Input: part model. Units: mm. Frame: model coordinates. Face numbers are marked on the shaded views. A direction names the side the tool comes from. Give positions to 0.01 mm unless a question says otherwise; leave off trailing zeros. Order: outer loops, then holes, each group sorted by start corner. A loop starts at its lowest first (then second) coordinate and runs counter-clockwise, first axis right, second up. Notation, with made-up numbers: (6.25, 1.25) -> (50.25, 1.25) arc R29 cw to (50.25, 29.25) -> close; hole circle Ø5 at (-30, -14). An arc over 180 degrees is marked (long way). Use a Markdown table: item, result. Add a question column.
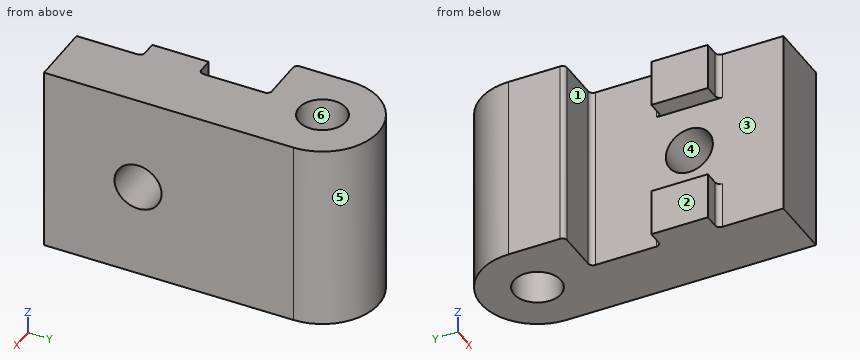
from build123d import *

# Parameters (mm, degrees)
SKETCH1_R           = 2.5
BOSS_EXTRUDE1_DEPTH = 20
SKETCH2_R           = 2.5
CUT_EXTRUDE1_DEPTH  = 20
SKETCH3_W           = 10
SKETCH3_H           = 6
CUT_EXTRUDE2_DEPTH  = 2
FILLET1_R           = 0.5
FILLET2_R           = 0.5


with BuildPart() as part:
    # Sketch1 → Boss-Extrude1 (new body)
    with BuildSketch(Plane.XY):
        with BuildLine():
            Line((6.3, -53.6), (6.3, -59.6))
            Line((6.3, -59.6), (7.3, -59.6))
            Line((7.3, -59.6), (8.3, -59.6))
            Line((8.3, -59.6), (8.3, -60.1))
            Line((8.3, -60.1), (8.3, -66.6))
            Line((8.3, -66.6), (15, -66.6))
            Line((15, -66.6), (15, -40.1))
            ThreePointArc((15, -40.1), (9, -34.1), (3, -40.1))
            Line((3, -40.1), (3, -46.1))
            Line((3, -46.1), (8.3, -46.1))
            Line((8.3, -46.1), (8.3, -46.6))
            Line((8.3, -46.6), (8.3, -53.1))
            Line((8.3, -53.1), (8.3, -53.6))
            Line((8.3, -53.6), (7.3, -53.6))
            Line((7.3, -53.6), (6.3, -53.6))
        make_face()
        with Locations((9, -40.1)):
            Circle(SKETCH1_R, mode=Mode.SUBTRACT)
    extrude(amount=BOSS_EXTRUDE1_DEPTH)

    # Sketch2 → Cut-Extrude1 (cut)
    with BuildSketch(Plane.ZY.offset(-6.3)):
        with Locations((10, -56.6)):
            Circle(SKETCH2_R)
    extrude(amount=-CUT_EXTRUDE1_DEPTH, mode=Mode.SUBTRACT)

    # Sketch3 → Cut-Extrude2 (cut)
    with BuildSketch(Plane.ZY.offset(-6.3)):
        with Locations((10, -56.6)):
            Rectangle(SKETCH3_W, SKETCH3_H)
    extrude(amount=-CUT_EXTRUDE2_DEPTH, mode=Mode.SUBTRACT)

    # Fillet1
    fillet1_edges = [part.edges().sort_by_distance(p)[0] for p in [
        (8.3, -46.1, 10),
        (3, -46.1, 10),
    ]]
    fillet(fillet1_edges, radius=FILLET1_R)

    # Fillet2
    fillet2_edges = [part.edges().sort_by_distance(p)[0] for p in [
        (8.3, -59.6, 17.5),
        (8.3, -53.6, 17.5),
        (8.3, -53.6, 2.5),
        (8.3, -59.6, 2.5),
    ]]
    fillet(fillet2_edges, radius=FILLET2_R)


solid = part.part
Q1. Section query A-A (x = 9). Return loops of the section in (y, z), plus the area to 3 significant figures.
Q2. Section query D-D (z = 17). Return loops of the section in (x, y), plus the area to 3 significant figures.
Q3. Section query B-B (z = 10). Return loops of the section in (x, y).
Q4. Access query for the marked faces 1, 2 and 3. Directions: +Z, -Z, +X, -X, +Y, -Y. A direction counts if a zero-diameter tool reaches every point of the face in a straight line with its end or side. Return the directions, or none.
Q5. Draft query along X for the marked faces 4, 5 and 6. Return one class per face: +X half, -X half, draft (parallel to the pull), parting line (faces both ways), or undercut.
Q6. First-contact query: pin 1 (1.5 mm diameter, centred on y = -58, z = 2, fed in from -X); pin 2 (1.7 mm diameter, centred on x = 7, z = 17, fed in from +Y); pin 3 (0.8 mm diameter, centred on x = 7.5, z = 16.5, fed in from -Y); pin 4 (4 mm diameter, centred on y = -56.6, z = 10, fed in from +X). Flat tips, straight axial feed; report the tip coordinate or a pass-through.
Q7. Ray query, line 1 (Y direction, x = 7.75, z = 1.75); line 2 (X direction, y = -40, z = 19); line 3 (Y direction, x = 9, z = 4.75). Return the intervals inside material, ascending.
Q8. Section query C-C (y = -56.6). Return loops of the section in (x, z), plus the area to 4 significant figures.
Solution:
| question | item | result |
|---|---|---|
| 1 | outline | (-66.6, 0) -> (-42.6, 0) -> (-42.6, 20) -> (-66.6, 20) -> close; (-37.6, 0) -> (-34.1, 0) -> (-34.1, 20) -> (-37.6, 20) -> close; hole circle Ø5 at (-56.6, 10) |
| 1 | area | 530 mm² |
| 2 | outline | (3, -45.6) arc R0.5 ccw to (3.5, -46.1) -> (7.8, -46.1) arc R0.5 cw to (8.3, -46.6) -> (8.3, -53.1) arc R0.5 cw to (7.8, -53.6) -> (6.3, -53.6) -> (6.3, -59.6) -> (7.8, -59.6) arc R0.5 cw to (8.3, -60.1) -> (8.3, -66.6) -> (15, -66.6) -> (15, -40.1) arc R6 ccw to (3, -40.1) -> close; hole circle Ø5 at (9, -40.1) |
| 2 | area | 258 mm² |
| 3 | outline | (3, -45.6) arc R0.5 ccw to (3.5, -46.1) -> (7.8, -46.1) arc R0.5 cw to (8.3, -46.6) -> (8.3, -54.1) -> (15, -54.1) -> (15, -40.1) arc R6 ccw to (3, -40.1) -> close; (8.3, -66.6) -> (15, -66.6) -> (15, -59.1) -> (8.3, -59.1) -> close; hole circle Ø5 at (9, -40.1) |
| 4 | face 1 | +Z, -Z, -X |
| 4 | face 2 | +Z, -Z, -X, -Y |
| 4 | face 3 | -X |
| 5 | face 4 | draft |
| 5 | face 5 | parting line |
| 5 | face 6 | undercut |
| 6 | pin 1 | stops at x = 6.3 |
| 6 | pin 2 | stops at y = -34.21 |
| 6 | pin 3 | stops at y = -59.61 |
| 6 | pin 4 | passes through |
| 7 | line 1 | y = -59.6 to -53.6, -46.1 to -42.27, -37.93 to -34.23 |
| 7 | line 2 | x = 3 to 6.5, 11.5 to 15 |
| 7 | line 3 | y = -66.6 to -42.6, -37.6 to -34.1 |
| 8 | outline | (6.3, 0) -> (15, 0) -> (15, 7.5) -> (8.3, 7.5) -> (8.3, 5) -> (6.3, 5) -> close; (6.3, 15) -> (8.3, 15) -> (8.3, 12.5) -> (15, 12.5) -> (15, 20) -> (6.3, 20) -> close |
| 8 | area | 120.5 mm² |
